from build123d import *

# Parameters (mm, degrees)
SKETCH1_R           = 2.5
SKETCH1_R_2         = 0.75
BOSS_EXTRUDE1_DEPTH = 2


with BuildPart() as part:
    # Sketch1 → Boss-Extrude1 (new body)
    with BuildSketch(Plane.XY):
        with Locations((-5.75, 0)):
            Circle(SKETCH1_R)
        with Locations((-5.75, 0)):
            Circle(SKETCH1_R_2, mode=Mode.SUBTRACT)
        with BuildLine():
            ThreePointArc((-4.905963303, 2.353211009), (-3.705483952, 1.438733515), (-3.25, 0))
            ThreePointArc((-3.25, 0), (-3.705483952, -1.438733515), (-4.905963303, -2.353211009))
            ThreePointArc((-4.905963303, -2.353211009), (0, -1.5), (4.905963303, -2.353211009))
            ThreePointArc((4.905963303, -2.353211009), (3.25, 0), (4.905963303, 2.353211009))
            ThreePointArc((4.905963303, 2.353211009), (0, 1.5), (-4.905963303, 2.353211009))
        make_face()
        with Locations((5.75, 0)):
            Circle(SKETCH1_R)
        with Locations((5.75, 0)):
            Circle(SKETCH1_R_2, mode=Mode.SUBTRACT)
    extrude(amount=BOSS_EXTRUDE1_DEPTH)


solid = part.part
The listing builds one solid part. Answer for the finished solid, in the listing's coordinates (mm). Round coordinates to 2 decimals unless told otherwise and drop trailing zeros. Write each loop counter-clockwise with the first axis right and the second up, starting at its lowest first coordinate (ties: lowest second). Pieces come first, ordered by that corner, then holes. Notation, with made-up numbers: M 3,57 L 20,57 A19 cw 20,81 Z; hole C 24,-24 d6. An arc over 180 degrees is marked long. Write each question's results on one line, items separated by ' | '. Start each with the question number.
Item 1: Find section B-B on y = 0. Write down the section's boundary in (x, z).
Item 2: Given pin 1 Ø1.4 at (x, y) = (5.75, 0) entering from +Z, flat-ended and moving along its own axis, determine where the tip first touches the part or whether it passes through.
Item 3: Find section D-D on y = 2.15. Write down the section's boundary in (x, z), and give its area (3 significant figures).
Item 4: Find section A-A on x = 5.75. Write down the section's boundary in (y, z), and give its area (3 significant figures).
Item 5: Find section C-C on z = 0.9. Write down the section's boundary in (x, y), and give its area (3 significant figures).
Item 6: The mould has two halves that part along X. Classify faces 1 (the flat face through (0, 0, 2)), 2 (the cylindrical face through (-0.1, -1.5, 1)): +X half, -X half, draft (parallel to the pull), parting line (faces both ways), or undercut.
Item 7: Straight lines are drawn through the part: probe 1 along Y at (x, z) = (-5.75, 0.5); probe 2 along X at (y, z) = (0.2, 1.75); probe 3 along Y at (x, z) = (-0.25, 1.7). For each, find the intervals that lie inside material, in ascending order.
Answer block:
1) outline: M -8.25,0 L -6.5,0 L -6.5,2 L -8.25,2 Z; M -5,0 L 5,0 L 5,2 L -5,2 Z; M 6.5,0 L 8.25,0 L 8.25,2 L 6.5,2 Z
2) pin 1: passes through
3) outline: M -7.03,0 L -4.3,0 L -4.3,2 L -7.03,2 Z; M 4.3,0 L 7.03,0 L 7.03,2 L 4.3,2 Z | area: 10.9 mm²
4) outline: M -2.5,0 L -0.75,0 L -0.75,2 L -2.5,2 Z; M 0.75,0 L 2.5,0 L 2.5,2 L 0.75,2 Z | area: 7.00 mm²
5) outline: M -4.91,-2.35 A14.53 cw 4.91,-2.35 A2.5 ccw long 4.91,2.35 A14.53 cw -4.91,2.35 A2.5 ccw long Z; hole C -5.75,0 d1.5; hole C 5.75,0 d1.5 | area: 59.3 mm²
6) face 1: draft | face 2: undercut
7) probe 1: y = -2.5 to -0.75, 0.75 to 2.5 | probe 2: x = -8.24 to -6.47, -5.03 to 5.03, 6.47 to 8.24 | probe 3: y = -1.5 to 1.5
